Autodesk Inventor part; units mm, degrees
ref_plane "YZ Plane" through (0, 0, 0) normal (1, 0, 0) x (0, 1, 0)
ref_plane "XZ Plane" through (0, 0, 0) normal (0, 1, 0) x (-1, 0, 0)
ref_plane "XY Plane" through (0, 0, 0) normal (0, 0, 1) x (1, 0, 0)
sketch "Sketch1" plane through (0, 0, 0) normal (0, 1, 0) x (-1, 0, 0)
  point P0 (0, 0)
sketch "Sketch2" plane through (0, 0, 0) normal (0, 1, 0) x (-1, 0, 0)
  line L0 (6.6745, 14.6831) -> (-112.3255, 14.6831)
  line L1 (-116.3255, 10.6831) -> (-116.3255, -62.3169)
  line L2 (-112.3255, -66.3169) -> (6.6745, -66.3169)
  line L3 (10.6745, -62.3169) -> (10.6745, 10.6831)
  arc A0 (10.6745, 10.6831) -> (6.6745, 14.6831) centre (6.6745, 10.6831) ccw
  arc A1 (6.6745, -66.3169) -> (10.6745, -62.3169) centre (6.6745, -62.3169) ccw
  arc A2 (-116.3255, -62.3169) -> (-112.3255, -66.3169) centre (-112.3255, -62.3169) ccw
  arc A3 (-112.3255, 14.6831) -> (-116.3255, 10.6831) centre (-112.3255, 10.6831) ccw
  point P0 (0, 0)
  point P1 (-116.3255, -66.3169)
  point P2 (-116.3255, 14.6831)
  point P3 (10.6745, -66.3169)
  dimension "d0" = 127
  dimension "d1" = 81
  dimension "d2" = 4
extrude "Extrusion1" add sketch "Sketch2" along normal blind 2
sketch "Sketch3" plane through (0, 2, 0) normal (0, 1, 0) x (1, 0, 0)
  line L0 (-10.6745, 62.3169) -> (-10.6745, -10.6831)
  line L1 (-10.6745, -10.6831) -> (-10.6745, -17.6831)
  line L2 (-10.6745, -17.6831) -> (-13.6745, -17.6831)
  line L3 (-5.6745, -17.6831) -> (111.3255, -17.6831)
  line L4 (119.3255, -9.6831) -> (119.3255, 61.3169)
  line L5 (111.3255, 69.3169) -> (-5.6745, 69.3169)
  line L6 (-13.6745, 61.3169) -> (-13.6745, -9.6831)
  arc A0 (-13.6745, -9.6831) -> (-5.6745, -17.6831) centre (-5.6745, -9.6831) ccw
  arc A1 (111.3255, -17.6831) -> (119.3255, -9.6831) centre (111.3255, -9.6831) ccw
  arc A2 (-5.6745, 69.3169) -> (-13.6745, 61.3169) centre (-5.6745, 61.3169) ccw
  arc A3 (119.3255, 61.3169) -> (111.3255, 69.3169) centre (111.3255, 61.3169) ccw
  point P0 (0, 0)
  point P1 (119.3255, 69.3169)
  point P2 (119.3255, -17.6831)
  point P3 (-13.6745, 69.3169)
  dimension "d5" = 7
  dimension "d6" = 3
  dimension "d7" = 133
  dimension "d8" = 87
  dimension "d9" = 8
  dimension "d10" = 8
extrude "Extrusion2" add sketch "Sketch3" along normal blind 3
fillet "Fillet1" radius 3 8 edges at (116.9823, 5, -66.9738) (52.8255, 5, -69.3169) (-11.3314, 5, -66.9738) (-13.6745, 5, -25.8169) (-11.3314, 5, 15.3399) (52.8255, 5, 17.6831) (116.9823, 5, 15.3399) (119.3255, 5, -25.8169)
fillet "Fillet2" radius 1 8 edges at (-9.503, 0, 13.5115) (-10.6745, 0, -25.8169) (-9.503, 0, -65.1453) (52.8255, 0, -66.3169) (115.1539, 0, -65.1453) (116.3255, 0, -25.8169) (115.1539, 0, 13.5115) (52.8255, 0, 14.6831)
properties part number "lid-v2"
Verification items for the finished model (mm, model axes). A direction names the side the tool comes from. Coordinates: 2 decimals unless noted, no trailing zeros. Order: outer loops, then holes, each group sorted by start corner. A loop starts at its lowest first (then second) coordinate and runs counter-clockwise, first axis right, second up. Notation, with made-up numbers: (-4, 20.25) -> (11, 20.25) arc R18 cw to (11, 38.25) -> close; hole circle Ø7 at (-28.5, -32). An arc over 180 degrees is marked (long way). Put each result on its own line as item: value. Start each with the question number.
1) Material ranges on L1, parallel to Z at x = 0.5, y = 1.35; L2, parallel to Z at x = 47.5, y = 2.35; L3, parallel to X at y = 0.4, z = -28, recorded low to high.
2) Cross-section at C-C (y = 3.75). Enter the section's corners in (x, z), plus the area to 3 significant figures.
3) Go/stop test with flat-tipped pins: pin 1 (0.5 mm diameter, centred on x = 71.5, y = 1.5, fed in from -Z); pin 2 (0.8 mm diameter, centred on x = 49, y = 1.5, fed in from +Z); pin 3 (1 mm diameter, centred on x = 9.5, y = 3.5, fed in from +Z). Record where each tip stops, or that it passes through.
4) Tool access check on faces 1 (the flat face through (53, 2, -68)), 2 (the cylindrical face through (-9.534, 1.493, -65.114)), 3 (the cylindrical face through (-9.472, 1.493, 13.542)). Record the directions out of +Z, -Z, +X, -X, +Y, -Y that give a thin tool (end or side, any length) a straight path to the whole face; none if there is none.
5) Release check for a two-part mould opening along Y. For faces 4 (the cylindrical face through (115.185, 1.493, 13.48)), 5 (the flat face through (54, 0, -25)), 6 (the cylindrical face through (53.644, 4.145, 16.781)) record: pulls with the +Y half, pulls with the -Y half, needs draft (parallel to the pull), parting line crosses it, or undercut.
Geometry check:
1. L1: z = -66.32 to 14.68
1. L2: z = -69.3 to 17.66
1. L3: x = -10.47 to 116.13
2. outline: (-13.11, -61.32) arc R7.44 ccw to (-5.67, -68.75) -> (111.33, -68.75) arc R7.44 ccw to (118.76, -61.32) -> (118.76, 9.68) arc R7.44 ccw to (111.33, 17.12) -> (-5.67, 17.12) arc R7.44 ccw to (-13.11, 9.68) -> close
2. area: 11,300 mm^2
3. pin 1: stops at z = -66.32
3. pin 2: stops at z = 14.68
3. pin 3: stops at z = 17.51
4. face 1: -Y
4. face 2: -Z, -X, -Y
4. face 3: +Z, -X, -Y
5. face 4: needs draft
5. face 5: pulls with the -Y half
5. face 6: pulls with the +Y half
